Can you work these out from the model? Positions are in its coordinate system, mm. Coordinates: 2 decimals unless noted, no trailing zeros. Order: outer loops, then holes, each group sorted by start corner. A loop starts at its lowest first (then second) coordinate and runs counter-clockwise, first axis right, second up. Notation, with made-up numbers: (78.5, 19.25) -> (129.5, 19.25) arc R15 cw to (129.5, 40.25) -> close; hole circle Ø3 at (-16.5, 65.5). An arc over 180 degrees is marked (long way). Answer in a Markdown table with one row per item.
```python
from build123d import *

# Parameters (mm, degrees)
F0_R     = 7.3025
F0_R_2   = 6.0325
F1_DEPTH = 0.635
F2_R     = 0.381
F3_R     = 7.3025
F3_R_2   = 2.4765
F4_DEPTH = 0.635


with BuildPart() as f1:
    # F0 (on Top) → F1 (new body)
    with BuildSketch(Plane.XY):
        Circle(F0_R)
        Circle(F0_R_2, mode=Mode.SUBTRACT)
    extrude(amount=F1_DEPTH)

    # F2
    f2_edges = [f1.edges().sort_by_distance(p)[0] for p in [
        (-7.3025, 0, 0.635),
        (-6.0325, 0, 0.635),
    ]]
    fillet(f2_edges, radius=F2_R)

    # F3 (on Top) → F4 (join)
    with BuildSketch(Plane.XY):
        Circle(F3_R)
        Circle(F3_R_2, mode=Mode.SUBTRACT)
    extrude(amount=-F4_DEPTH)


solid = f1.part
```
(1) I need wall thicknesses on line 1 (Y direction, x = 0, z = -0.35); line 2 (Z direction, x = -0.75, y = -2.5) (3 decimals); line 3 (X direction, y = 3.25, z = 0.3). Which ranges of each line are inside material? Lowest first, please. Write a range as [from, to].
Response values:
| item | result |
|---|---|
| line 1 | [-7.3, -2.48], [2.48, 7.3] |
| line 2 | [-0.635, 0] |
| line 3 | [-6.54, -5.09], [5.09, 6.54] |
(2) We'd pull the mould along X, two halves only. Please class faces 1 (the cylindrical face through (-0.322, 2.455, -0.313)), 2 (the flat face through (0, -3, 0)), 3 (the flat face through (3, 0, -0.635)), 4 (the cylindrical face through (-5.38, 4.94, -0.18)): +X half, -X half, draft (parallel to the pull), parting line (faces both ways), or undercut.
Response values:
| item | result |
|---|---|
| face 1 | undercut |
| face 2 | undercut |
| face 3 | draft |
| face 4 | parting line |
(3) Suppose I cut it at C-C (z = 0.45). Please give me the cut outline in (x, y).
Response values:
| item | result |
|---|---|
| outline | circle Ø14.5 at (0, 0); hole circle Ø12.17 at (0, 0) |
(4) Will this pin go through, and if not, where does the flat tip stop? pin 1 Ø3 at (x, y) = (-2.5, -2.5) entering from +Z.
Response values:
| item | result |
|---|---|
| pin 1 | z = 0 |
